```python
from build123d import *

# Parameters (mm, degrees)
SKETCH1_W           = 100
SKETCH1_H           = 72.5
BOSS_EXTRUDE1_DEPTH = 10
CUT_EXTRUDE1_DEPTH  = 10
SKETCH3_W           = 100
SKETCH3_H           = 10
FEET_DEPTH          = 20
SKETCH4_R           = 3
FEET_HOLE_DEPTH     = 10
SKETCH6_W           = 8
SKETCH6_H           = 15
BOSS_EXTRUDE2_DEPTH = 18
CUT_EXTRUDE2_DEPTH  = 105.485644947
SKETCH5_R           = 4
SKETCH5_R_2         = 10
CUT_EXTRUDE3_DEPTH  = 9.8
FILLET1_R           = 5
FILLET2_R           = 15


with BuildPart() as part:
    # Sketch1 → Boss-Extrude1 (new body)
    with BuildSketch(Plane.XY):
        with Locations((50, 36.25)):
            Rectangle(SKETCH1_W, SKETCH1_H)
    extrude(amount=BOSS_EXTRUDE1_DEPTH)

    # Sketch2 → Cut-Extrude1 (cut)
    with BuildSketch(Plane.XY.offset(10)):
        with BuildLine():
            Line((85, 65), (85, 72.5))
            Line((85, 72.5), (15, 72.5))
            Line((15, 72.5), (15, 65))
            ThreePointArc((15, 65), (50, 30), (85, 65))
        make_face()
    extrude(amount=-CUT_EXTRUDE1_DEPTH, mode=Mode.SUBTRACT)

    # Sketch3 → feet (add)
    with BuildSketch(Plane.XY.offset(10)):
        with Locations((50, 5)):
            Rectangle(SKETCH3_W, SKETCH3_H)
    extrude(amount=FEET_DEPTH)

    # Sketch4 → feet-hole (cut)
    with BuildSketch(Plane.XZ):
        with Locations(Location((20, 20, 0), (0, 0, 270))):
            Circle(SKETCH4_R)
        with Locations(Location((80, 20, 0), (0, 0, 270))):
            Circle(SKETCH4_R)
        with Locations(Location((50, 20, 0), (0, 0, 270))):
            Circle(SKETCH4_R)
    extrude(amount=-FEET_HOLE_DEPTH, mode=Mode.SUBTRACT)

    # Sketch6 → Boss-Extrude2 (add)
    with BuildSketch(Plane.XY.offset(10)):
        with Locations((35, 17.5)):
            Rectangle(SKETCH6_W, SKETCH6_H)
        with Locations((65, 17.5)):
            Rectangle(SKETCH6_W, SKETCH6_H)
    extrude(amount=BOSS_EXTRUDE2_DEPTH)

    # Sketch7 → Cut-Extrude2 (cut, through all)
    with BuildSketch(Plane.ZY.offset(-31)):
        Polygon((10, 25), (28, 10), (28, 25), align=None)
    extrude(amount=-CUT_EXTRUDE2_DEPTH, mode=Mode.SUBTRACT)

    # Sketch5 → Cut-Extrude3 (cut)
    with BuildSketch(Plane.XY.offset(10)):
        with Locations((7.5, 65)):
            Circle(SKETCH5_R)
        with Locations(Location((92.5, 65, 0), (0, 0, 180))):
            Circle(SKETCH5_R)
        with Locations((15, 25)):
            Circle(SKETCH5_R_2)
        with Locations(Location((85, 25, 0), (0, 0, 180))):
            Circle(SKETCH5_R_2)
    extrude(amount=-CUT_EXTRUDE3_DEPTH, mode=Mode.SUBTRACT)

    # Fillet1
    fillet1_edges = [part.edges().sort_by_distance(p)[0] for p in [
        (0, 72.5, 5),
        (15, 72.5, 5),
        (85, 72.5, 5),
        (100, 72.5, 5),
    ]]
    fillet(fillet1_edges, radius=FILLET1_R)

    # Fillet2
    fillet2_edges = [part.edges().sort_by_distance(p)[0] for p in [
        (0, 5, 30),
        (100, 5, 30),
    ]]
    fillet(fillet2_edges, radius=FILLET2_R)


solid = part.part
```
Part model, mm, in its own coordinate system. A direction names the side the tool comes from. Give positions to 0.01 mm unless a question says otherwise; leave off trailing zeros. Write each loop counter-clockwise with the first axis right and the second up, starting at its lowest first coordinate (ties: lowest second). Pieces come first, ordered by that corner, then holes. Notation, with made-up numbers: (60, 21.5) -> (98, 21.5) arc R18 ccw to (98, 55.5) -> close; hole circle Ø11 at (63, 49.25). An arc over 180 degrees is marked (long way). Put each result on its own line as item: value. Start each with the question number.
Item 1: Wall check: L1, parallel to X at y = 67, z = 7; L2, parallel to X at y = 6.25, z = 20; L3, parallel to Z at x = 88, y = 35. Give the ranges that are in metal, low to high. Write a range as [from, to].
Item 2: Cut at D-D (y = 6). List the corners of the cut face in (x, z), then the cut area to 3 significant figures.
Item 3: Which spindle directions (+Z, -Z, +X, -X, +Y, -Y) get a long thin tool onto all of the face, cutting with end or side? Do faces 4 (the face through (69, 16, 17)), 5 (the face through (15, 25, 0.2)), 6 (the face through (15, 66, 5)), 7 (the face through (61, 16, 17)), 8 (the face through (1.43, 71, 5.07)). Say none if no direction does.
Item 4: Cut at B-B (z = 3.5). List the corners of the cut face in (x, y), then the cut area to 3 significant figures.
Item 5: Cut at A-A (x = 50). List the corners of the cut face in (y, z).
Item 6: Pin check, flat tips, straight feed: pin 1 Ø6.5 at (x, y) = (92.5, 65) entering from +Z; pin 2 Ø5 at (x, z) = (80, 20) entering from -Y; pin 3 Ø16.5 at (y, z) = (19, 19) entering from -X; pin 4 Ø1 at (y, z) = (17, 11.5) entering from +X. Stop position of each tip, or through.
Item 7: Cut at C-C (y = 41). List the corners of the cut face in (x, z).
Item 8: Pull direction Z, two halves, no side cores. Call faces 1 (the face through (24.54, 28, 5.17)), 2 (the face through (18.2, 4.9, 22.4)), 3 (the face through (4.28, 5.07, 25.49)): pulls with the +Z half, pulls with the -Z half, needs draft (parallel to the pull), parting line crosses it, or undercut.
Answer list:
1. L1: x = [0, 4.04], [10.96, 15], [85, 89.04], [95.96, 100]
1. L2: x = [0.86, 17], [23, 47], [53, 77], [83, 99.14]
1. L3: z = [0, 10]
2. outline: (0, 0) -> (100, 0) -> (100, 15) arc R15 ccw to (85, 30) -> (15, 30) arc R15 ccw to (0, 15) -> close; hole circle Ø6 at (20, 20); hole circle Ø6 at (50, 20); hole circle Ø6 at (80, 20)
2. area: 2,820 mm2
3. face 4: +Z, +X, +Y
3. face 5: +Z
3. face 6: +Z, -Z, +Y
3. face 7: +Z, +Y
3. face 8: +Z, -Z, -X, +Y
4. outline: (0, 0) -> (100, 0) -> (100, 67.5) arc R5 ccw to (95, 72.5) -> (90, 72.5) arc R5 ccw to (85, 67.5) -> (85, 65) arc R35 cw to (15, 65) -> (15, 67.5) arc R5 ccw to (10, 72.5) -> (5, 72.5) arc R5 ccw to (0, 67.5) -> close; hole circle Ø8 at (7.5, 65); hole circle Ø20 at (15, 25); hole circle Ø20 at (85, 25); hole circle Ø8 at (92.5, 65)
4. area: 4,050 mm2
5. outline: (0, 0) -> (30, 0) -> (30, 10) -> (10, 10) -> (10, 17) -> (0, 17) -> close; (0, 23) -> (10, 23) -> (10, 30) -> (0, 30) -> close
6. pin 1: stops at z = 0.2
6. pin 2: passes through
6. pin 3: stops at x = 31
6. pin 4: stops at x = 69
7. outline: (0, 0) -> (24.52, 0) -> (24.52, 10) -> (0, 10) -> close; (75.48, 0) -> (100, 0) -> (100, 10) -> (75.48, 10) -> close
8. face 1: needs draft
8. face 2: undercut
8. face 3: pulls with the +Z half
